from build123d import *

# Parameters (mm, degrees)
BOSS_EXTRUDE1_DEPTH = 1.6
SKETCH2_W           = 6.615656004
SKETCH2_H           = 7.718265338
SKETCH2_W_2         = 10.396030864
SKETCH2_H_2         = 12.364976103
BOSS_EXTRUDE2_DEPTH = 10.8
SKETCH3_R           = 1.5875
CUT_EXTRUDE1_DEPTH  = 2.6


with BuildPart() as part:
    # Sketch1 → Boss-Extrude1 (new body)
    with BuildSketch(Plane(origin=(0, 0, 0), x_dir=(1, 0, 0), z_dir=(0, 1, 0))):
        Polygon((0, 68.58), (0, 2.54), (2.5, 2.54), (5.04, 0), (38.04, 0), (40.58, 2.54), (53.34, 2.54), (53.34, 68.58), align=None)
    extrude(amount=BOSS_EXTRUDE1_DEPTH)

    # Sketch2 → Boss-Extrude2 (add)
    with BuildSketch(Plane(origin=(0, 1.6, 0), x_dir=(1, 0, 0), z_dir=(0, 1, 0))):
        with Locations((7.533094465, 65.806229304)):
            Rectangle(SKETCH2_W, SKETCH2_H)
        with Locations((38.642429245, 68.129584686)):
            Rectangle(SKETCH2_W_2, SKETCH2_H_2)
    extrude(amount=BOSS_EXTRUDE2_DEPTH)

    # Sketch3 → Cut-Extrude1 (cut, through all)
    with BuildSketch(Plane(origin=(0, 1.6, 0), x_dir=(1, 0, 0), z_dir=(0, 1, 0))):
        with Locations((7.62, 2.54)):
            Circle(SKETCH3_R)
        with Locations((35.56, 2.54)):
            Circle(SKETCH3_R)
        with Locations((50.8, 53.34)):
            Circle(SKETCH3_R)
        with Locations((2.54, 54.61)):
            Circle(SKETCH3_R)
    extrude(amount=-CUT_EXTRUDE1_DEPTH, mode=Mode.SUBTRACT)


solid = part.part
Check sheet for the modelled part. Datum: model origin and axes. Units: mm. A direction names the side the tool comes from. Round coordinates to 2 decimals unless told otherwise and drop trailing zeros. Order: outer loops, then holes, each group sorted by start corner. A loop starts at its lowest first (then second) coordinate and runs counter-clockwise, first axis right, second up.
(1) Cross-section at A-A, the plane x = 35.56. Enter the section's corners in (y, z), and give its area (3 significant figures).
(2) Cross-section at B-B, the plane y = 5.75. Enter the section's corners in (x, z), and give its area (3 significant figures).
(3) Draft check along Z on faces 5 (the flat face through (39, 7, -61.947)), 6 (the flat face through (53.34, 1, -35)), 7 (the cylindrical face through (2.2, 0.81, -53.06)). Enter one of: pulls with the +Z half, pulls with the -Z half, needs draft (parallel to the pull), parting line crosses it, or undercut.
(4) Access from +Z, -Z, +X, -X, +Y, -Y to the whole of each face (thin tool, end or side, straight path). Record for faces 1 (the flat face through (47, 1, -2.54)), 2 (the flat face through (10.841, 7, -66)), 3 (the flat face through (7, 7, -69.665)), 4 (the flat face through (27, 1, -68.58)).
(5) Go/stop test with flat-tipped pins: P1, Ø5, axis at x = 7.62, z = -2.54, coming from the -Y side; P2, Ø1.9, axis at x = 2.54, z = -54.61, coming from the +Y side; P3, Ø4, axis at y = 5.5, z = -67.5, coming from the +X side; P4, Ø1.5, axis at x = 35.5, z = -48, coming from the +Y side. Record where each tip stops, or that it passes through.
(6) Scan lines: probe 1 along Z at (x, y) = (50.8, 0.55); probe 2 along X at (y, z) = (6, -64); probe 3 along X at (y, z) = (0.5, -54.61). Record each from-to range of solid material in increasing order.
(7) Cross-section at C-C, the plane x = 7.62. Enter the section's corners in (y, z).
(8) Cross-section at D-D, the plane z = -21.5. Enter the section's corners in (x, y).
Check sheet entries:
1. outline: (0, -68.58) - (1.6, -68.58) - (1.6, -74.31) - (12.4, -74.31) - (12.4, -61.95) - (1.6, -61.95) - (1.6, -4.13) - (0, -4.13) - close; (0, -0.95) - (1.6, -0.95) - (1.6, 0) - (0, 0) - close
1. area: 238 mm2
2. outline: (4.23, -69.67) - (10.84, -69.67) - (10.84, -61.95) - (4.23, -61.95) - close; (33.44, -74.31) - (43.84, -74.31) - (43.84, -61.95) - (33.44, -61.95) - close
2. area: 180 mm2
3. face 5: pulls with the +Z half
3. face 6: needs draft
3. face 7: undercut
4. face 1: +Z, +X, +Y, -Y
4. face 2: +Z, -Z, +Y
4. face 3: -Z, -X, +Y, -Y
4. face 4: -Z, +X, -X, -Y
5. P1: stops at y = 0
5. P2: passes through
5. P3: stops at x = 43.84
5. P4: stops at y = 1.6
6. probe 1: z = -68.58 to -54.93, -51.75 to -2.54
6. probe 2: x = 4.23 to 10.84, 33.44 to 43.84
6. probe 3: x = 0 to 0.95, 4.13 to 49.85, 51.75 to 53.34
7. outline: (0, -68.58) - (1.6, -68.58) - (1.6, -69.67) - (12.4, -69.67) - (12.4, -61.95) - (1.6, -61.95) - (1.6, -4.13) - (0, -4.13) - close; (0, -0.95) - (1.6, -0.95) - (1.6, 0) - (0, 0) - close
8. outline: (0, 0) - (53.34, 0) - (53.34, 1.6) - (0, 1.6) - close
